Work out the finished part from the listing and answer in its coordinate system (mm). Give positions to 0.01 mm unless a question says otherwise; leave off trailing zeros. Write each loop counter-clockwise with the first axis right and the second up, starting at its lowest first coordinate (ties: lowest second). Pieces come first, ordered by that corner, then holes.
1) Straight lines are drawn through the part: probe 1 along X at (y, z) = (-40, 0.4); probe 2 along X at (y, z) = (-5.5, 1.15); probe 3 along X at (y, z) = (-1.5, 1.15). For each, find the intervals that lie inside material, in ascending order.
2) Find section B-B (x = 43.5). Determine the outline of the cut face in (y, z).
3) Given pin 1 Ø1.6 at (x, y) = (1.778, -4.318) entering from +Z, flat-ended and moving along its own axis, determine where the tip first touches the part or whether it passes through.
4) Find section A-A (x = 1). Determine the outline of the cut face in (y, z), plus the area to 3 significant figures.
5) Determine the mould class of faces 1 (the face through (23, 0, 1)), 2 (the face through (45.013, -3.497, 1.014)), 3 (the face through (23, -22, 0)) for opening direction Y: pulls with the +Y half, pulls with the -Y half, needs draft (parallel to the pull), parting line crosses it, or undercut.
Autodesk Fusion 360 part; units mm, degrees
sketch "Sketch10" plane through (0, 0, 0) normal (0, 0, 1) x (1, 0, 0)
  line L0 (0, 0) -> (45.72, 0)
  arc A0 (48.26, -2.54) -> (45.72, 0) centre (45.72, -2.54) ccw
  line L1 (45.72, -2.54) -> (48.26, -2.54) construction
  line L2 (45.72, -2.54) -> (45.72, 0) construction
  line L3 (48.26, -2.54) -> (48.26, -42.4361)
  arc A1 (48.26, -2.54) -> (45.72, 0) centre (45.72, -2.54) ccw
  arc A2 (45.72, -44.9761) -> (48.26, -42.4361) centre (45.72, -42.4361) ccw
  line L4 (0, -42.4361) -> (-2.54, -42.4361) construction
  line L5 (45.72, -44.9761) -> (0, -44.9761)
  arc A3 (-2.54, -42.4361) -> (0, -44.9761) centre (0, -42.4361) ccw
  arc A4 (-2.54, -42.4361) -> (0, -44.9761) centre (0, -42.4361) ccw
  line L6 (0, -42.4361) -> (0, -44.9761) construction
  arc A5 (0, 0) -> (-2.54, -2.54) centre (0, -2.54) ccw
  line L7 (-2.54, -42.4361) -> (-2.54, -2.54)
  point P0 (45.72, -44.9761)
  dimension "d5" = 45.72
  dimension "d7" = 2.54
  dimension "d8" = 90
  dimension "d9" = 39.8961
  dimension "d10" = 2.54
  dimension "d11" = 2.54
  dimension "d12" = 45.72
  dimension "d13" = 2.54
  dimension "d14" = 90
  dimension "d15" = 39.8961
  dimension "d16" = 2.54
  dimension "d17" = 2.54
extrude "Extrude3" add sketch "Sketch10" along normal blind 2
sketch "Sketch11" plane through (0, 0, 2) normal (0, 0, 1) x (-1, 0, 0)
  arc A0 (-45.72, 44.9761) -> (-48.26, 42.4361) centre (-45.72, 42.4361) ccw
  line L0 (-48.26, 42.4361) -> (-48.26, 2.54)
  arc A1 (-48.26, 2.54) -> (-45.72, 0) centre (-45.72, 2.54) ccw
  line L1 (-45.72, 0) -> (0, 0)
  arc A2 (0, 0) -> (2.54, 2.54) centre (0, 2.54) ccw
  line L2 (2.54, 2.54) -> (2.54, 42.4361)
  arc A3 (2.54, 42.4361) -> (0, 44.9761) centre (0, 42.4361) ccw
  line L3 (0, 44.9761) -> (-45.72, 44.9761)
  circle A4 centre (-1.778, 4.318) radius 1.35
  dimension "d22" = 2.7
extrude "Extrude4" cut sketch "Sketch11" against normal blind 4 contours A4
sketch "Sketch12" plane through (0, 0, 2) normal (0, 0, 1) x (-1, 0, 0)
  circle A0 centre (-1.778, 4.318) radius 1.35
  arc A1 (-45.72, 44.9761) -> (-48.26, 42.4361) centre (-45.72, 42.4361) ccw
  line L0 (-48.26, 42.4361) -> (-48.26, 2.54)
  arc A2 (-48.26, 2.54) -> (-45.72, 0) centre (-45.72, 2.54) ccw
  line L1 (-45.72, 0) -> (0, 0)
  arc A3 (0, 0) -> (2.54, 2.54) centre (0, 2.54) ccw
  line L2 (2.54, 2.54) -> (2.54, 42.4361)
  arc A4 (2.54, 42.4361) -> (0, 44.9761) centre (0, 42.4361) ccw
  line L3 (0, 44.9761) -> (-45.72, 44.9761)
  circle A5 centre (-43.942, 4.318) radius 1.35
  dimension "d27" = 2.7
extrude "Extrude5" cut sketch "Sketch12" against normal blind 4 contours A5
sketch "Sketch13" plane through (0, 0, 2) normal (0, 0, 1) x (-1, 0, 0)
  circle A0 centre (-43.942, 4.318) radius 1.35
  circle A1 centre (-1.778, 4.318) radius 1.35
  arc A2 (-45.72, 44.9761) -> (-48.26, 42.4361) centre (-45.72, 42.4361) ccw
  line L0 (-48.26, 42.4361) -> (-48.26, 2.54)
  arc A3 (-48.26, 2.54) -> (-45.72, 0) centre (-45.72, 2.54) ccw
  line L1 (-45.72, 0) -> (0, 0)
  arc A4 (0, 0) -> (2.54, 2.54) centre (0, 2.54) ccw
  line L2 (2.54, 2.54) -> (2.54, 42.4361)
  arc A5 (2.54, 42.4361) -> (0, 44.9761) centre (0, 42.4361) ccw
  line L3 (0, 44.9761) -> (-45.72, 44.9761)
  circle A6 centre (-1.778, 40.6581) radius 1.35
  dimension "d32" = 2.7
extrude "Extrude6" cut sketch "Sketch13" against normal blind 4 contours A6
sketch "Sketch14" plane through (0, 0, 2) normal (0, 0, 1) x (-1, 0, 0)
  circle A0 centre (-1.778, 40.6581) radius 1.35
  circle A1 centre (-43.942, 4.318) radius 1.35
  circle A2 centre (-1.778, 4.318) radius 1.35
  arc A3 (-45.72, 44.9761) -> (-48.26, 42.4361) centre (-45.72, 42.4361) ccw
  line L0 (-48.26, 42.4361) -> (-48.26, 2.54)
  arc A4 (-48.26, 2.54) -> (-45.72, 0) centre (-45.72, 2.54) ccw
  line L1 (-45.72, 0) -> (0, 0)
  arc A5 (0, 0) -> (2.54, 2.54) centre (0, 2.54) ccw
  line L2 (2.54, 2.54) -> (2.54, 42.4361)
  arc A6 (2.54, 42.4361) -> (0, 44.9761) centre (0, 42.4361) ccw
  line L3 (0, 44.9761) -> (-45.72, 44.9761)
  circle A7 centre (-43.942, 40.6581) radius 1.35
  dimension "d37" = 2.7
extrude "Extrude7" cut sketch "Sketch14" against normal blind 4 contours A7
sketch "Sketch15" plane through (0, 0, 2) normal (0, 0, 1) x (-1, 0, 0)
  circle A0 centre (-43.942, 40.6581) radius 1.35
  circle A1 centre (-1.778, 40.6581) radius 1.35
  circle A2 centre (-43.942, 4.318) radius 1.35
  circle A3 centre (-1.778, 4.318) radius 1.35
  arc A4 (-45.72, 44.9761) -> (-48.26, 42.4361) centre (-45.72, 42.4361) ccw
  line L0 (-48.26, 42.4361) -> (-48.26, 2.54)
  arc A5 (-48.26, 2.54) -> (-45.72, 0) centre (-45.72, 2.54) ccw
  line L1 (-45.72, 0) -> (0, 0)
  arc A6 (0, 0) -> (2.54, 2.54) centre (0, 2.54) ccw
  line L2 (2.54, 2.54) -> (2.54, 42.4361)
  arc A7 (2.54, 42.4361) -> (0, 44.9761) centre (0, 42.4361) ccw
  line L3 (0, 44.9761) -> (-45.72, 44.9761)
  line L4 (-4.96, 7.5) -> (-40.76, 7.5)
  line L5 (-40.76, 7.5) -> (-40.76, 37.4761)
  line L6 (-40.76, 37.4761) -> (-4.96, 37.4761)
  line L7 (-4.96, 37.4761) -> (-4.96, 7.5)
Results:
1. probe 1: x = -2.54 to 0.6, 2.96 to 42.76, 45.12 to 48.26
1. probe 2: x = -2.54 to 1.13, 2.43 to 43.29, 44.59 to 48.26
1. probe 3: x = -2.32 to 48.04
2. outline: (-44.98, 0) - (-41.93, 0) - (-41.93, 2) - (-44.98, 2) - close; (-39.38, 0) - (-5.59, 0) - (-5.59, 2) - (-39.38, 2) - close; (-3.04, 0) - (0, 0) - (0, 2) - (-3.04, 2) - close
3. pin 1: passes through
4. outline: (-44.98, 0) - (-41.76, 0) - (-41.76, 2) - (-44.98, 2) - close; (-39.55, 0) - (-5.42, 0) - (-5.42, 2) - (-39.55, 2) - close; (-3.21, 0) - (0, 0) - (0, 2) - (-3.21, 2) - close
4. area: 81.1 mm2
5. face 1: pulls with the +Y half
5. face 2: undercut
5. face 3: needs draft
